Read the model definition and answer for the solid it produces. Units are mm, in the model's axes. A direction names the side the tool comes from. Coordinates: 2 decimals unless noted, no trailing zeros. Write each loop counter-clockwise with the first axis right and the second up, starting at its lowest first coordinate (ties: lowest second). Pieces come first, ordered by that corner, then holes.
Autodesk Inventor part; units mm, degrees
ref_plane "YZ Plane" through (0, 0, 0) normal (1, 0, 0) x (0, 1, 0)
ref_plane "XZ Plane" through (0, 0, 0) normal (0, 1, 0) x (-1, 0, 0)
ref_plane "XY Plane" through (0, 0, 0) normal (0, 0, 1) x (1, 0, 0)
sketch "スケッチ1" plane through (0, 0, 0) normal (0, 1, 0) x (-1, 0, 0)
  circle A0 centre (0, 0) radius 1.15
  circle A1 centre (0, 0) radius 2
  circle A2 centre (0, 0) radius 2.9
  line L0 (-2, 0) -> (2, 0)
  line L1 (2, 0) -> (2, -2.9)
  line L2 (2, -2.9) -> (-2, -2.9)
  line L3 (-2, -2.9) -> (-2, 0)
  line L4 (0, 0) -> (0, 2.9)
  line L5 (0, 0) -> (2.9, 0)
  line L6 (2.9, 0) -> (2.9, 10)
  line L7 (2.9, 10) -> (0, 10)
  line L8 (0, 10) -> (0, 0)
  point P0 (0, 2)
  point P1 (2, -2.1)
  point P2 (-2, -2.1)
  dimension "d1" = 4
  dimension "d2" = 5.8
  dimension "d0" = 2.3
  dimension "d3" = 10
extrude "押し出し1" add sketch "スケッチ1" along normal blind 4.5 contours L5 A2 L1 | A1 L4 A2 L5 | A2 L8 L7 L6
extrude "押し出し2" add sketch "スケッチ1" along normal blind 3.5 contours A1 L3 A2 L4
extrude "押し出し3" add sketch "スケッチ1" against normal blind 1 contours L0 A1 A0 | A0 L4 A1 L0 | A0 L0 A1 L4 | L1 A2 L3 A1 | L5 A2 L1 | A1 L4 A2 L5 | A1 L3 A2 L4 | A2 L8 L7 L6
sketch "スケッチ2" plane through (-2.9, 4.5, 10) normal (0, 0, 1) x (1, 0, 0)
  line L0 (2.9, -4.5) -> (1.4, -4.5)
  line L1 (1.4, -4.5) -> (1.4, -4)
  line L2 (1.4, -4) -> (2.9, -4)
  line L3 (2.9, -4) -> (2.9, -4.5)
  dimension "d10" = 1.5
  dimension "d11" = 0.5
hole "穴1" at (-1.5, 0.5, 10) direction (0, 0, -1) diameter 1 end through all
sketch "スケッチ3" plane through (-2.9, 4.5, 10) normal (0, 0, 1) x (1, 0, 0)
  line L0 (0.9, 0) -> (0, 0)
  line L1 (0, 0) -> (4, 0)
  line L2 (4, 0) -> (4, -4)
  line L3 (4, -4) -> (0, -4)
  line L4 (0, -4) -> (0, 0)
  line L5 (0, 0) -> (3.25, 0)
  line L6 (3.25, 0) -> (3.25, -3.25)
  line L7 (3.25, -3.25) -> (0, -3.25)
  line L8 (0, -3.25) -> (0, 0)
  line L9 (0, 0) -> (1.625, 0)
  line L10 (1.625, 0) -> (1.625, -1.625)
  line L11 (1.625, -1.625) -> (0, -1.625)
  line L12 (0, -1.625) -> (0, 0)
  line L13 (0, -3.25) -> (4, -3.25)
  line L14 (4, -3.25) -> (4, 0.75)
  line L15 (4, 0.75) -> (0, 0.75)
  line L16 (0, 0.75) -> (0, -3.25)
  point P0 (2.9, -4.5)
  dimension "d19" = 4
  dimension "d20" = 4
  dimension "d21" = 3.25
  dimension "d22" = 3.25
  dimension "d33" = 4
  dimension "d34" = 4
extrude "押し出し4" add sketch "スケッチ3" along normal blind 10 and the other way blind 3 contours L1 L10 L11 L4 L0 | L0 L16 L15 L14 L1 | L1 L6 L7 L4 L11 L10 | L1 L2 L13 L6
chamfer "面取り1" distance 0.75 angle 45 1 edges at (-0.9, 5.25, 7)
chamfer "面取り2" distance 1.1 angle 45 1 edges at (1.1, 2.8752, 7)
sketch "スケッチ6" plane through (-2.9, 4.5, 20) normal (0, 0, 1) x (1, 0, 0)
  line L0 (0, 0) -> (0, 0.75)
  line L1 (0, 0.75) -> (2, 0.75)
  line L2 (2, 0.75) -> (2, -1.25)
  line L3 (2, -1.25) -> (0, -1.25)
  line L4 (0, -1.25) -> (0, 0.75)
  circle A0 centre (2, -1.25) radius 1.1
  point P0 (2.9, -4.5)
  dimension "d41" = 2
  dimension "d42" = 2
  dimension "d43" = 2.2
extrude "押し出し6" cut sketch "スケッチ6" against normal blind 10 contours A0 L2 L3 | L3 L2 A0
properties part number "srod1.6right"
Item 1: The part is cut by section C-C (x = -2.5). Give the vertices of the cut face in (y, z).
Item 2: Find the intervals of material crossed by probe 1 along X at (y, z) = (3.25, 17.75); probe 2 along X at (y, z) = (-0.3, 0); probe 3 along Y at (x, z) = (-1.5, 8), in increasing order.
Item 3: For faces 5 (the flat face through (2, 3.5, 1)), 6 (the flat face through (-2, 4.5, 4)), 7 (the flat face through (0, 0, -2)), determine the directions among +Z, -Z, +X, -X, +Y, -Y from which every point of the face is accessible in a straight line to the end or side of a thin tool.
Item 4: Determine the mould class of faces 1 (the flat face through (-2.9, 2, 10)), 2 (the cylindrical face through (-1.711, 3.993, 15.07)), 3 (the cylindrical face through (2.775, 1.1, -0.843)), 4 (the flat face through (2, 2, -1)) for opening direction X: +X half, -X half, draft (parallel to the pull), parting line (faces both ways), or undercut.
Item 5: Given pin 1 (2.5 mm diameter, centred on y = 2, z = -1.5, fed in from +X); pin 2 (3 mm diameter, centred on y = 2.5, z = 16, fed in from +X); pin 3 (1.1 mm diameter, centred on x = -2, y = -0.5, fed in from +Z); pin 4 (3 mm diameter, centred on x = -0.9, y = 3.25, fed in from +Z), each flat-ended and moving along its own axis, determine where each tip first touches the part or whether it passes through.
Item 6: The part is cut by section A-A (z = 15.5). Give the vertices of the cut face in (x, y), and give its area (3 significant figures).
Item 7: The part is cut by section D-D (z = 5.75). Give the vertices of the cut face in (x, y), and give its area (3 significant figures).
Answer:
1. outline: (-1, -1.47) - (4.5, -1.47) - (4.5, 7) - (5.25, 7.75) - (5.25, 20) - (1.25, 20) - (1.25, 10) - (-1, 10) - close
2. probe 1: x = -2.9 to -2, 0.2 to 1.1
2. probe 2: x = -2.9 to -1.15, 1.15 to 2.9
2. probe 3: y = -1 to 0, 1 to 5.25
3. face 5: -Z, +X, +Y
3. face 6: -Z, +X, -X, +Y
3. face 7: -Z, +Y
4. face 1: -X half
4. face 2: undercut
4. face 3: parting line
4. face 4: undercut
5. pin 1: stops at x = 2.89
5. pin 2: stops at x = 1.1
5. pin 3: stops at z = 10
5. pin 4: stops at z = 20
6. outline: (-2.9, 1.25) - (1.1, 1.25) - (1.1, 5.25) - (-2.9, 5.25) - close; hole circle Ø2.2 at (-0.9, 3.25)
6. area: 12.2 mm2
7. outline: (-2.9, -1) - (0, -1) - (0, 4.5) - (-2.9, 4.5) - close; hole circle Ø1 at (-1.5, 0.5)
7. area: 15.2 mm2
